Autodesk Inventor part; units mm, degrees
ref_plane "Work Plane1" through (25, 0, 0) normal (1, 0, 0) x (0, 1, 0)
ref_plane "XZ Plane" through (0, 0, 0) normal (0, 1, 0) x (-1, 0, 0)
ref_plane "XY Plane" through (0, 0, 0) normal (0, 0, 1) x (1, 0, 0)
sketch "Sketch1" plane through (0, 0, 0) normal (0, 0, 1) x (1, 0, 0)
  circle A0 centre (0, 0) radius 5
  dimension "d0" = 10
extrude "Extrusion1" add sketch "Sketch1" along normal blind 20
sketch "Sketch2" plane through (0, 0, 20) normal (0, 0, 1) x (1, 0, 0)
  circle A0 centre (0, 0) radius 5
hole "Hole1" at (0, 0, 20) direction (0, 0, -1) diameter 6 depth 8
ref_plane "Work Plane1" through (25, 0, 0) normal (1, 0, 0) x (0, 1, 0)
sketch "Sketch3" plane through (25, 0, 0) normal (1, 0, 0) x (0, 1, 0)
  circle A0 centre (0, 10) radius 3
  line L0 (-5, 0) -> (-5, 20)
  point P0 (0, 0)
  point P1 (-5, 10)
  dimension "d11" = 6
extrude "Extrusion2" add sketch "Sketch3" against normal up to surface
thread "Thread1"
properties part number "verbindungunten"
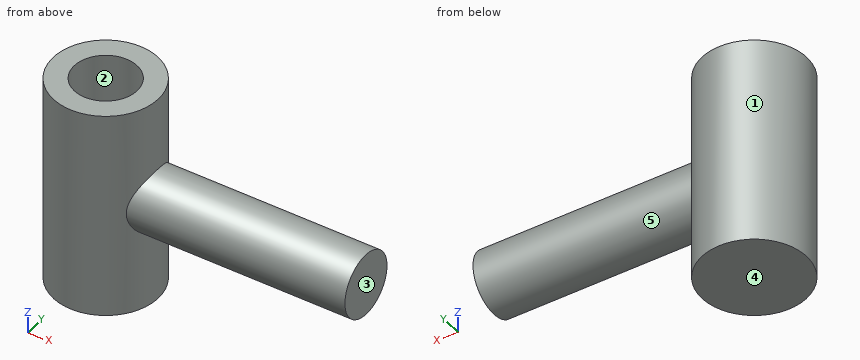
The model under review builds one solid part; all positions refer to its coordinate system, in mm. Face numbers are marked on the shaded views. A direction names the side the tool comes from. Give positions to 0.01 mm unless a question says otherwise; leave off trailing zeros. Write each loop counter-clockwise with the first axis right and the second up, starting at its lowest first coordinate (ties: lowest second). Pieces come first, ordered by that corner, then holes. Notation, with made-up numbers: M 20.25,28.5 L 57.25,28.5 A22 ccw 57.25,44.5 Z; hole C -35.75,-26.75 d1. An arc over 180 degrees is marked long. Answer in a Markdown table with one row per item.
Item 1: Add section A-A on y = 0. Give the boundary of the cut face in (x, z), plus the area to 3 significant figures.
Check sheet entries:
| item | result |
|---|---|
| outline | M -5,0 L 5,0 L 5,7 L 25,7 L 25,13 L 5,13 L 5,20 L 3,20 L 3,12 L -3,12 L -3,20 L -5,20 Z |
| area | 272 mm2 |
Item 2: Add section B-B on x = 0. Give the boundary of the cut face in (y, z).
Check sheet entries:
| item | result |
|---|---|
| outline | M -5,0 L 5,0 L 5,20 L 3,20 L 3,12 L -3,12 L -3,20 L -5,20 Z |
Item 3: For P1, Ø5, axis at x = 6.5, z = 2, coming from the -Y side; P2, Ø1.5, axis at y = -2, z = 9.5, coming from the -X side, all flat-tipped, find the tip position at first contact; note any pin that passes through.
Check sheet entries:
| item | result |
|---|---|
| P1 | y = -3 |
| P2 | x = -4.84 |
Item 4: For line 1 along Y through (x, z) = (0, 16.75); line 2 along X through (y, z) = (4, 15.5); line 3 along Z through (x, y) = (1.5, -2.25), list the stretches that pass through material, from the lowest coordinate up.
Check sheet entries:
| item | result |
|---|---|
| line 1 | -5 to -3, 3 to 5 |
| line 2 | -3 to 3 |
| line 3 | 0 to 12 |
Item 5: Add section D-D on z = 10. Give the boundary of the cut face in (x, y), plus the area to 3 significant figures.
Check sheet entries:
| item | result |
|---|---|
| outline | M 4,-3 L 25,-3 L 25,3 L 4,3 A5 ccw long Z |
| area | 200 mm2 |
Item 6: Add section C-C on z = 17.5. Give the boundary of the cut face in (x, y), plus the area to 3 significant figures.
Check sheet entries:
| item | result |
|---|---|
| outline | C 0,0 d10; hole C 0,0 d6 |
| area | 50.3 mm2 |
Item 7: Draft analysis for pull direction Y (two halves, no side actions). For the marked faces 1, 2 and 3, state which applies: +Y half, -Y half, draft (parallel to the pull), parting line (faces both ways), or undercut.
Check sheet entries:
| item | result |
|---|---|
| face 1 | parting line |
| face 2 | undercut |
| face 3 | draft |
Item 8: Tool access review of the marked faces 4 and 5: name each direction out of +Z, -Z, +X, -X, +Y, -Y from which nothing blocks a thin tool from reaching the whole face with its end or side.
Check sheet entries:
| item | result |
|---|---|
| face 4 | -Z, +X, -X, +Y, -Y |
| face 5 | +X |
